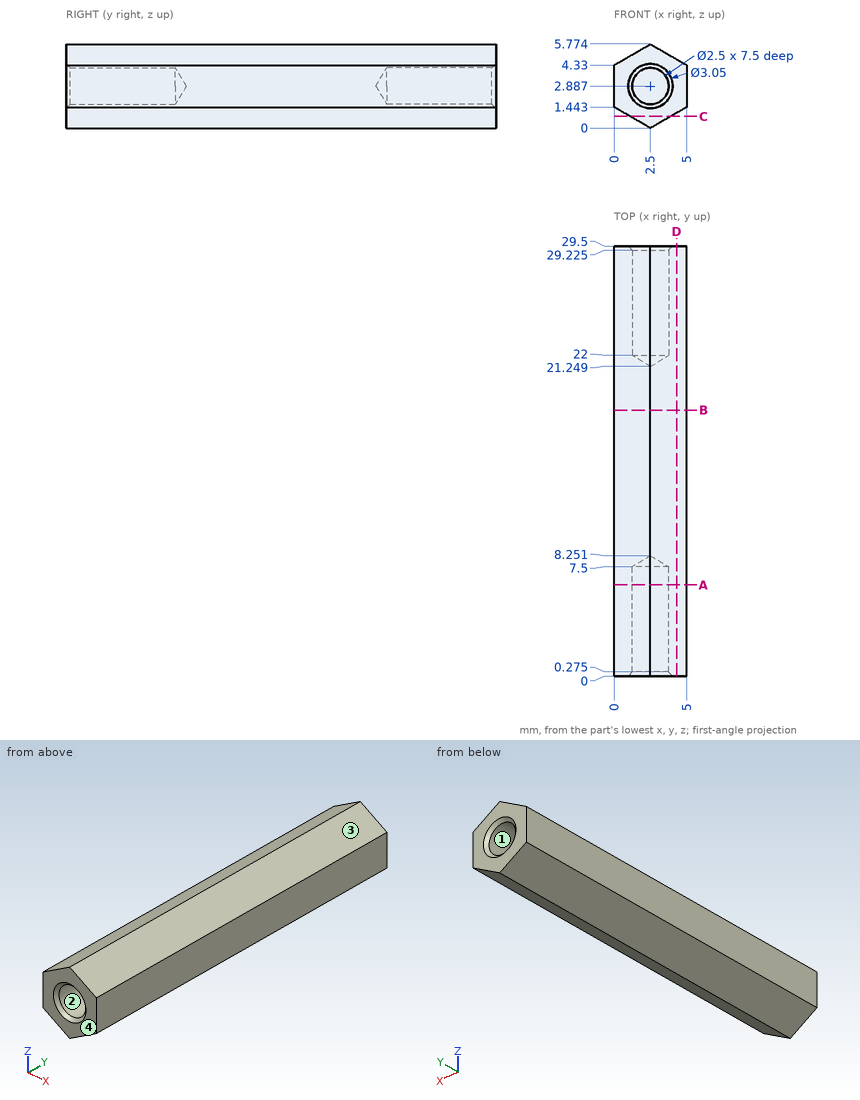
Can you work these out from the drawing? Everything is in mm from the part's minimum corner. Give positions to 0.01 mm unless a question says otherwise; leave off trailing zeros. Loops run counter-clockwise (first coordinate to the right, second up) from the corner with the lowest first, then second, coordinate; pieces in that order, holes last. Notation, with made-up numbers: (58.25, 81) -> (85.25, 81) arc R12 ccw to (85.25, 95) -> close; hole circle Ø3 at (-23.5, -15.5). An arc over 180 degrees is marked (long way). Write item = value, one per line.
1) I need wall thicknesses on L1, parallel to Y at x = 3.35, z = 4.15 (1 decimal); L2, parallel to Z at x = 3.25, y = 25.5 (1 decimal); L3, parallel to Z at x = 4.85, y = 6 (1 decimal). Which ranges of each line are inside material? Lowest first, please. Write a range as from..to.
Check result:
L1 = 0..29.5
L2 = 0.4..1.9, 3.9..5.3
L3 = 1.4..4.4
2) Suppose I cut it at B-B on y = 18.25. Write out the boundary of the cut face in (x, z).
Check result:
outline = (0, 1.44) -> (2.5, 0) -> (5, 1.44) -> (5, 4.33) -> (2.5, 5.77) -> (0, 4.33) -> close
3) Thinking about a two-plate mould opening in Z: for the marked faces 1, 2, 3 and 4, which applies, released by +Z, released by -Z, zero draft, split by the parting line, or undercut?
Check result:
face_1 = undercut
face_2 = undercut
face_3 = released by +Z
face_4 = zero draft
4) Will these pins go through, and if not, where does the flat tip stop? pin 1 (1.5 mm diameter, centred on x = 3.5, y = 9.5, fed in from -Z) (1 decimal); pin 2 (1.5 mm diameter, centred on x = 2.5, z = 2.89, fed in from -Y); pin 3 (2 mm diameter, centred on x = 1, y = 25.5, fed in from +Z) (1 decimal).
Check result:
pin_1 = 0.1
pin_2 = 7.8
pin_3 = 5.5
5) Suppose I cut it at D-D on x = 4.3. Write out the boundary of the cut face in (y, z) (1 decimal).
Check result:
outline = (0, 1) -> (29.5, 1) -> (29.5, 4.7) -> (0, 4.7) -> close
6) Suppose I cut it at A-A on y = 6.25. Write out the boundary of the cut face in (x, z).
Check result:
outline = (0, 1.44) -> (2.5, 0) -> (5, 1.44) -> (5, 4.33) -> (2.5, 5.77) -> (0, 4.33) -> close; hole circle Ø2.5 at (2.5, 2.89)
7) Suppose I cut it at C-C on z = 0.8. Write out the boundary of the cut face in (x, y) (1 decimal).
Check result:
outline = (1.1, 0) -> (3.9, 0) -> (3.9, 29.5) -> (1.1, 29.5) -> close
